The listing builds one solid part. Answer for the finished solid, in the listing's coordinates (mm). A direction names the side the tool comes from. Coordinates: 2 decimals unless noted, no trailing zeros. Loops run counter-clockwise (first coordinate to the right, second up) from the corner with the lowest first, then second, coordinate; pieces in that order, holes last. Notation, with made-up numbers: M 19.25,81.5 L 29.25,81.5 A18 ccw 29.25,116.5 Z; hole C 32.5,-31 d4. An arc over 180 degrees is marked long. Return JSON: item names as keys, results as strings. Group by question number.
1. Section B-B (x = 15.25) is taken. Write down the section's boundary in (y, z), then the cut area to 3 significant figures.
2. Section C-C (z = 1.7) is taken. Write down the section's boundary in (x, y).
3. Which of the six approach directions +Z, -Z, +X, -X, +Y, -Y give full straight-line access (tool end or side, diameter ignored) to faces 1 (the face through (-1.27, -0.97, 3.48)), 2 (the face through (15, -3, 1))?
4. Straight lines are drawn through the part: L1, parallel to X at y = 0, z = 4.4; L2, parallel to Y at x = 15, z = 3.7; L3, parallel to X at y = -0.5, z = 1.05. For each, find the intervals that lie inside material, in ascending order. Write a range as from..to.
5. Section A-A (z = 3.35) is taken. Write down the section's boundary in (x, y), then the cut area to 3 significant figures.
6. Given P1, Ø5, axis at x = -1.5, y = 0, coming from the -Z side; P2, Ø2.5, axis at x = 9.5, z = 2, coming from the -Y side; P3, Ø2.5, axis at x = 15, y = 0, coming from the +Z side; P4, Ø2, axis at x = 0, z = 1, coming from the -Y side, each flat-ended and moving along its own axis, determine where each tip first touches the part or whether it passes through.
7. The mould has two halves that part along Y. Classify faces 3 (the face through (12.4, -1.5, 1)), 4 (the face through (-4, 0, 2)), 5 (the face through (8, 0, 0)), 6 (the face through (-2.6, -1.5, 1)): pulls with the +Y half, pulls with the -Y half, needs draft (parallel to the pull), parting line crosses it, or undercut.
8. Section D-D (y = 2) is taken. Write down the section's boundary in (x, z), then the cut area to 3 significant figures.
```python
from build123d import *

# Parameters (mm, degrees)
SKETCH1_R           = 1.6
BOSS_EXTRUDE1_DEPTH = 5
CUT_EXTRUDE1_DEPTH  = 2


with BuildPart() as part:
    # Sketch1 → Boss-Extrude1 (new body)
    with BuildSketch(Plane.XY):
        with BuildLine():
            Line((0, 4), (15, 4))
            ThreePointArc((15, 4), (19, 0), (15, -4))
            Line((15, -4), (7, -4))
            ThreePointArc((7, -4), (3.5, -7.5), (0, -4))
            ThreePointArc((0, -4), (-4, 0), (0, 4))
        make_face()
        Circle(SKETCH1_R, mode=Mode.SUBTRACT)
        with Locations((15, 0)):
            Circle(SKETCH1_R, mode=Mode.SUBTRACT)
    extrude(amount=BOSS_EXTRUDE1_DEPTH)

    # Sketch2 → Cut-Extrude1 (cut)
    with BuildSketch(Plane(origin=(0, 0, 0), x_dir=(-1, 0, 0), z_dir=(0, 0, -1))):
        Polygon((3.464101615, 0), (1.732050808, 3), (-1.732050808, 3), (-3.464101615, 0), (-1.732050808, -3), (1.732050808, -3), align=None)
        Polygon((-11.535898385, 0), (-13.267949192, 3), (-16.732050808, 3), (-18.464101615, 0), (-16.732050808, -3), (-13.267949192, -3), align=None)
    extrude(amount=-CUT_EXTRUDE1_DEPTH, mode=Mode.SUBTRACT)


solid = part.part
```
Worked out:
{
 "1": {"outline": "M -3.99,0 L -3,0 L -3,2 L -1.58,2 L -1.58,5 L -3.99,5 Z; M 1.58,2 L 3,2 L 3,0 L 3.99,0 L 3.99,5 L 1.58,5 Z", "area": "18.4 mm^2"},
 "2": {"outline": "M 0,-4 A3.5 ccw 7,-4 L 15,-4 A4 ccw 15,4 L 0,4 A4 ccw Z; hole M -3.46,0 L -1.73,-3 L 1.73,-3 L 3.46,0 L 1.73,3 L -1.73,3 Z; hole M 11.54,0 L 13.27,-3 L 16.73,-3 L 18.46,0 L 16.73,3 L 13.27,3 Z"},
 "3": {"face 1": "+Z, -Z", "face 2": "-Z"},
 "4": {"L1": "-4..-1.6, 1.6..13.4, 16.6..19", "L2": "-4..-1.6, 1.6..4", "L3": "-3.97..-3.18, 3.18..11.82, 18.18..18.97"},
 "5": {"outline": "M 0,-4 A3.5 ccw 7,-4 L 15,-4 A4 ccw 15,4 L 0,4 A4 ccw Z; hole C 0,0 d3.2; hole C 15,0 d3.2", "area": "173 mm^2"},
 "6": {"P1": "z = 0", "P2": "y = -4", "P3": "through", "P4": "y = -6.45"},
 "7": {"face 3": "undercut", "face 4": "parting line crosses it", "face 5": "needs draft", "face 6": "undercut"},
 "8": {"outline": "M -3.46,0 L -2.31,0 L -2.31,2 L 2.31,2 L 2.31,0 L 12.69,0 L 12.69,2 L 17.31,2 L 17.31,0 L 18.46,0 L 18.46,5 L -3.46,5 Z", "area": "91.2 mm^2"}
}
